Work out the finished part from the listing and answer in its coordinate system (mm). A direction names the side the tool comes from. Give positions to 0.01 mm unless a question says otherwise; leave off trailing zeros. Write each loop counter-clockwise with the first axis right and the second up, starting at its lowest first coordinate (ties: lowest second). Pieces come first, ordered by that corner, then holes.
1) Given pin 1 Ø1 at (y, z) = (4.5, 4) entering from +X; pin 2 Ø4.5 at (y, z) = (-15, 14.9) entering from -X; pin 3 Ø6.5 at (x, y) = (-30, 15) entering from -Z, each flat-ended and moving along its own axis, determine where each tip first touches the part or whether it passes through.
2) Find section A-A (y = 15). Determine the outline of the cut face in (x, z), plus the area to 3 significant figures.
3) A tool of negligible diameter and unlimited length cuts with its end or side. For faces 1 (the face through (2.5, 15.1, 7.3)), 2 (the face through (50, 0, 17)), from which of +Z, -Z, +X, -X, +Y, -Y can it reach the whole face along a straight path? Write none if from no direction.
4) Straight lines are drawn through the part: probe 1 along Y at (x, z) = (18, 14.75); probe 2 along X at (y, z) = (15, 3.5); probe 3 along X at (y, z) = (15, 8.5). For each, find the intervals that lie inside material, in ascending order.
5) Find section D-D (x = -30). Determine the outline of the cut face in (y, z).
6) Find section B-B (x = -16). Determine the outline of the cut face in (y, z).
7) Determine the mould class of faces 3 (the face through (-27.5, 15.1, 7.3)), 4 (the face through (1, 23, 1)), 5 (the face through (48, 0, 1)), 6 (the face through (32.5, 15.1, 7.3)) for opening direction X: pulls with the +X half, pulls with the -X half, needs draft (parallel to the pull), parting line crosses it, or undercut.
8) Find section C-C (y = -15). Determine the outline of the cut face in (x, z).
```python
from build123d import *

# Parameters (mm, degrees)
SKETCH1_W               = 100
SKETCH1_H               = 50
BOSS_EXTRUDE1_DEPTH     = 30
SKETCH2_R               = 2.5
CUT_EXTRUDE1_DEPTH      = 108.354552768
FILLET1_R               = 5
CUT_EXTRUDE2_REACH      = 65.443
CUT_EXTRUDE2_END_RADIUS = 2.5
SKETCH3_R               = 2.5
FILLET2_R               = 5


with BuildPart() as part:
    # Sketch1 → Boss-Extrude1 (new body)
    with BuildSketch(Plane.XY):
        Rectangle(SKETCH1_W, SKETCH1_H)
    extrude(amount=BOSS_EXTRUDE1_DEPTH)

    # Sketch2 → Cut-Extrude1 (cut, through all)
    with BuildSketch(Plane(origin=(50, 0, 0), x_dir=(0, 0, -1), z_dir=(1, 0, 0))):
        with Locations(Location((-14.903548917, 15, 0), (0, 0, 90))):
            Circle(SKETCH2_R)
        with Locations(Location((-14.903548917, -15, 0), (0, 0, 90))):
            Circle(SKETCH2_R)
    extrude(amount=-CUT_EXTRUDE1_DEPTH, mode=Mode.SUBTRACT)

    # Fillet1
    fillet1_edges = [part.edges().sort_by_distance(p)[0] for p in [
        (0, -25, 0),
        (-50, 0, 0),
        (0, 25, 0),
        (50, 0, 0),
    ]]
    fillet(fillet1_edges, radius=FILLET1_R)

    # Cut-Extrude2: up to this cylinder (the profile starts outside it)
    cut_extrude2_end = Plane(origin=(0, 15, 14.903548917), z_dir=(1, 0, 0)) * Cylinder(CUT_EXTRUDE2_END_RADIUS, 196.886, mode=Mode.PRIVATE)
    # Sketch3 → Cut-Extrude2 (cut, up to the surface)
    with BuildSketch(Plane(origin=(0, 0, 0), x_dir=(-1, 0, 0), z_dir=(0, 0, -1)), mode=Mode.PRIVATE) as cut_extrude2_sk1:
        with Locations((-30, 15)):
            Circle(SKETCH3_R)
    cut_extrude2_tool1 = extrude(cut_extrude2_sk1.sketch, amount=-CUT_EXTRUDE2_REACH, mode=Mode.PRIVATE) - cut_extrude2_end
    add(cut_extrude2_tool1.solids().sort_by_distance((30, 15, 0))[0], mode=Mode.SUBTRACT)
    # Sketch3 → Cut-Extrude2 (cut, up to the surface)
    with BuildSketch(Plane(origin=(0, 0, 0), x_dir=(-1, 0, 0), z_dir=(0, 0, -1)), mode=Mode.PRIVATE) as cut_extrude2_sk2:
        with Locations((30, 15)):
            Circle(SKETCH3_R)
    cut_extrude2_tool2 = extrude(cut_extrude2_sk2.sketch, amount=-CUT_EXTRUDE2_REACH, mode=Mode.PRIVATE) - cut_extrude2_end
    add(cut_extrude2_tool2.solids().sort_by_distance((-30, 15, 0))[0], mode=Mode.SUBTRACT)
    # Sketch3 → Cut-Extrude2 (cut, up to the surface)
    with BuildSketch(Plane(origin=(0, 0, 0), x_dir=(-1, 0, 0), z_dir=(0, 0, -1)), mode=Mode.PRIVATE) as cut_extrude2_sk3:
        with Locations((0, 15)):
            Circle(SKETCH3_R)
    cut_extrude2_tool3 = extrude(cut_extrude2_sk3.sketch, amount=-CUT_EXTRUDE2_REACH, mode=Mode.PRIVATE) - cut_extrude2_end
    add(cut_extrude2_tool3.solids().sort_by_distance((0, 15, 0))[0], mode=Mode.SUBTRACT)

    # Fillet2
    # the kernel refuses this fillet: 5 mm, written as the material it takes off along each edge
    with BuildSketch(Plane(origin=(-45, -20, 5), x_dir=(0, -1, 0), z_dir=(-1, 0, 0))) as fillet2_piece_1_section:
        Polygon((0, 0), (FILLET2_R, 0), (FILLET2_R, -FILLET2_R), (0, -FILLET2_R), align=None)
    fillet2_piece_1 = extrude(amount=FILLET2_R, mode=Mode.PRIVATE)
    fillet2_piece_1 = fillet2_piece_1 - Plane(origin=(-45, -20, 5), x_dir=(0, 0.7071067811865475, 0.7071067811865475), z_dir=(-1, 0, 0)) * Sphere(FILLET2_R, mode=Mode.PRIVATE)
    add(fillet2_piece_1, mode=Mode.SUBTRACT)
    with BuildSketch(Plane(origin=(-45, 20, 5), x_dir=(-1, 0, 0), z_dir=(0, 1, 0))) as fillet2_piece_2_section:
        Polygon((0, 0), (FILLET2_R, 0), (FILLET2_R, -FILLET2_R), (0, -FILLET2_R), align=None)
    fillet2_piece_2 = extrude(amount=FILLET2_R, mode=Mode.PRIVATE)
    fillet2_piece_2 = fillet2_piece_2 - Plane(origin=(-45, 20, 5), x_dir=(0.7071067811865475, 0, 0.7071067811865475), z_dir=(0, 1, 0)) * Sphere(FILLET2_R, mode=Mode.PRIVATE)
    add(fillet2_piece_2, mode=Mode.SUBTRACT)
    with BuildSketch(Plane(origin=(45, -20, 5), x_dir=(0, -1, 0), z_dir=(1, 0, 0))) as fillet2_piece_3_section:
        Polygon((0, 0), (FILLET2_R, 0), (FILLET2_R, FILLET2_R), (0, FILLET2_R), align=None)
    fillet2_piece_3 = extrude(amount=FILLET2_R, mode=Mode.PRIVATE)
    fillet2_piece_3 = fillet2_piece_3 - Plane(origin=(45, -20, 5), x_dir=(0, 0.7071067811865475, 0.7071067811865475), z_dir=(1, 0, 0)) * Sphere(FILLET2_R, mode=Mode.PRIVATE)
    add(fillet2_piece_3, mode=Mode.SUBTRACT)
    with BuildSketch(Plane(origin=(45, 20, 5), x_dir=(1, 0, 0), z_dir=(0, 1, 0))) as fillet2_piece_4_section:
        Polygon((0, 0), (FILLET2_R, 0), (FILLET2_R, FILLET2_R), (0, FILLET2_R), align=None)
    fillet2_piece_4 = extrude(amount=FILLET2_R, mode=Mode.PRIVATE)
    fillet2_piece_4 = fillet2_piece_4 - Plane(origin=(45, 20, 5), x_dir=(-0.7071067811865475, 0, 0.7071067811865475), z_dir=(0, 1, 0)) * Sphere(FILLET2_R, mode=Mode.PRIVATE)
    add(fillet2_piece_4, mode=Mode.SUBTRACT)
    with BuildSketch(Plane(origin=(50, -25, 5), x_dir=(0, 1, 0), z_dir=(0, 0, 1)), Plane(origin=(50, 25, 5), x_dir=(-1, 0, 0), z_dir=(0, 0, 1))) as fillet2_piece_5:
        with BuildLine():
            CenterArc((FILLET2_R, FILLET2_R), FILLET2_R, 180, 90)
            Line((0, FILLET2_R), (0, 0))
            Line((0, 0), (FILLET2_R, 0))
        make_face()
    extrude(amount=37.5, mode=Mode.SUBTRACT)
    with BuildSketch(Plane(origin=(-50, -25, 5), x_dir=(0, 1, 0), z_dir=(0, 0, 1)), Plane(origin=(-50, 25, 5), x_dir=(1, 0, 0), z_dir=(0, 0, 1))) as fillet2_piece_6:
        with BuildLine():
            CenterArc((FILLET2_R, -FILLET2_R), FILLET2_R, 90, 90)
            Line((0, -FILLET2_R), (0, 0))
            Line((0, 0), (FILLET2_R, 0))
        make_face()
    extrude(amount=37.5, mode=Mode.SUBTRACT)


solid = part.part
```
Results:
1. pin 1: stops at x = 49.97
1. pin 2: passes through
1. pin 3: stops at z = 0
2. outline: (-50, 5) arc R5 ccw to (-45, 0) - (-32.5, 0) - (-32.5, 12.4) - (-50, 12.4) - close; (-50, 17.4) - (50, 17.4) - (50, 30) - (-50, 30) - close; (-27.5, 0) - (-2.5, 0) - (-2.5, 12.4) - (-27.5, 12.4) - close; (2.5, 0) - (27.5, 0) - (27.5, 12.4) - (2.5, 12.4) - close; (32.5, 0) - (45, 0) arc R5 ccw to (50, 5) - (50, 12.4) - (32.5, 12.4) - close
2. area: 2,300 mm2
3. face 1: -Z
3. face 2: +Z, -Z, +X, +Y, -Y
4. probe 1: y = -25 to -17.5, -12.5 to 12.5, 17.5 to 25
4. probe 2: x = -49.77 to -32.5, -27.5 to -2.5, 2.5 to 27.5, 32.5 to 49.77
4. probe 3: x = -50 to -32.5, -27.5 to -2.5, 2.5 to 27.5, 32.5 to 50
5. outline: (-25, 5) arc R5 ccw to (-20, 0) - (12.5, 0) - (12.5, 14.9) arc R2.5 cw to (17.5, 14.9) - (17.5, 0) - (20, 0) arc R5 ccw to (25, 5) - (25, 30) - (-25, 30) - close; hole circle Ø5 at (-15, 14.9)
6. outline: (-25, 5) arc R5 ccw to (-20, 0) - (20, 0) arc R5 ccw to (25, 5) - (25, 30) - (-25, 30) - close; hole circle Ø5 at (-15, 14.9); hole circle Ø5 at (15, 14.9)
7. face 3: undercut
7. face 4: needs draft
7. face 5: pulls with the +X half
7. face 6: undercut
8. outline: (-50, 5) arc R5 ccw to (-45, 0) - (45, 0) arc R5 ccw to (50, 5) - (50, 12.4) - (-50, 12.4) - close; (-50, 17.4) - (50, 17.4) - (50, 30) - (-50, 30) - close
